Geometry: final body of the model. Coordinates: model frame, mm. Face numbers are marked on the shaded views. A direction names the side the tool comes from. Give positions to 0.01 mm unless a question says otherwise; leave off trailing zeros. Order: outer loops, then holes, each group sorted by start corner. A loop starts at its lowest first (then second) coordinate and runs counter-clockwise, first axis right, second up. Notation, with made-up numbers: (62, 81) -> (91, 81) arc R18 ccw to (91, 85) -> close; hole circle Ø5 at (82.25, 72.25). An arc over 180 degrees is marked (long way). One line per question, with ' | ' between items. Start each with the question number.
(1) Section C-C (y = -5.25). Return loops of the section in (x, z).
(2) Ray query, L1, parallel to Y at x = 0, z = 1.15; L2, parallel to Y at x = 4.5, z = 4.1; L3, parallel to Z at x = 0, y = -5.5. Return the intervals inside material, ascending.
(3) First-contact query: pin 1 Ø1.7 at (x, z) = (0, 4) entering from -Y; pin 2 Ø1.3 at (x, y) = (-2.5, -6) entering from +Z. Flat tips, straight axial feed; report the tip coordinate or a pass-through.
(4) Section D-D (z = 2.6). Return loops of the section in (x, y).
(5) Set-up query: the marked faces 1, 2 and 3. Return all of +Z, -Z, +X, -X, +Y, -Y with unobstructed straight access to the full face (end or side cutting, diameter ignored); none if empty.
(6) Section B-B (x = -3.25). Return loops of the section in (y, z), then the cut area to 3 significant figures.
(7) Mould query, pull axis Y, two halves, no side actions, for the marked faces 4, 5 and 6. Classes: +Y half, -Y half, draft (parallel to the pull), parting line (faces both ways), or undercut.
(8) Section A-A (z = 1.4). Return loops of the section in (x, y).
```python
from build123d import *

# Parameters (mm, degrees)
F0_W     = 10.8
F0_H     = 9.4
F1_DEPTH = 4.4
F3_DEPTH = 10.8
F4_R     = 0.5


with BuildPart() as f1:
    # F0 (on Top) → F1 (new body)
    with BuildSketch(Plane.XY):
        Rectangle(F0_W, F0_H)
    extrude(amount=F1_DEPTH)

    # F2 (on face) → F3 (join, through all)
    with BuildSketch(Plane(origin=(-5.4, 0, 0), x_dir=(0, -1, 0), z_dir=(-1, 0, 0))):
        Polygon((7.799318, 2.9), (4.7, 2.9), (4.7, 2.4), (7.4, 2.4), (7.799318, 2.4), align=None)
        Polygon((7.799318, 0.581989), (7.799318, 2.4), (7.4, 2.4), (7.4, 0.281082), align=None)
        Polygon((9.799318, 0.300908), (7.799318, 0.581989), (7.4, 0.281082), (9.4, 0), align=None)
        Polygon((11.940386, 0), (9.799318, 0.300908), (9.4, 0), align=None)
    extrude(amount=-F3_DEPTH)

    # F4
    f4_edges = [f1.edges().sort_by_distance(p)[0] for p in [
        (0, -7.799318, 2.9),
        (0, -7.4, 2.4),
        (0, -7.4, 0.281082),
        (0, -7.799318, 0.581989),
    ]]
    fillet(f4_edges, radius=F4_R)


solid = f1.part
```
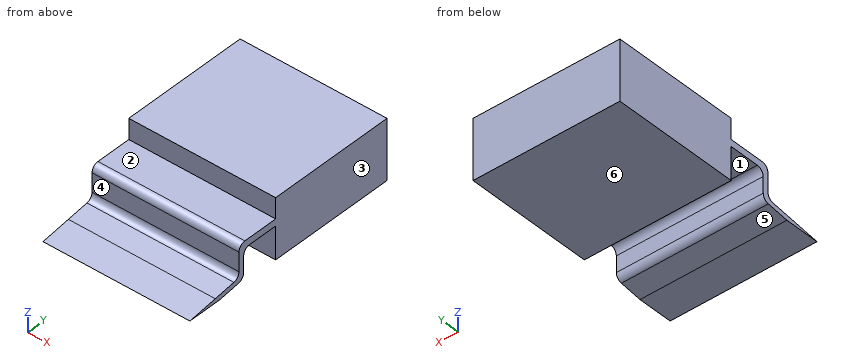
Response:
1) outline: (-5.4, 2.4) -> (5.4, 2.4) -> (5.4, 2.9) -> (-5.4, 2.9) -> close
2) L1: y = -7.8 to -7.4, -4.7 to 4.7 | L2: y = -4.7 to 4.7 | L3: z = 2.4 to 2.9
3) pin 1: stops at y = -4.7 | pin 2: stops at z = 2.9
4) outline: (-5.4, -7.76) -> (5.4, -7.76) -> (5.4, 4.7) -> (-5.4, 4.7) -> close
5) face 1: -Z, +X, -X | face 2: +Z, +X, -X, -Y | face 3: +Z, -Z, +X, +Y, -Y
6) outline: (-11.94, 0) -> (-9.4, 0) -> (-7.83, 0.22) arc R0.5 ccw to (-7.4, 0.72) -> (-7.4, 1.9) arc R0.5 cw to (-6.9, 2.4) -> (-4.7, 2.4) -> (-4.7, 0) -> (4.7, 0) -> (4.7, 4.4) -> (-4.7, 4.4) -> (-4.7, 2.9) -> (-7.3, 2.9) arc R0.5 ccw to (-7.8, 2.4) -> (-7.8, 1.02) arc R0.5 cw to (-8.23, 0.52) -> (-9.8, 0.3) -> close | area: 44.8 mm^2
7) face 4: -Y half | face 5: undercut | face 6: draft
8) outline: (-5.4, -7.8) -> (5.4, -7.8) -> (5.4, -7.4) -> (-5.4, -7.4) -> close; (-5.4, -4.7) -> (5.4, -4.7) -> (5.4, 4.7) -> (-5.4, 4.7) -> close
